from build123d import *

# Parameters (mm, degrees)
F2_DEPTH = 7.5
F3_DEPTH = 10


with BuildPart() as f2:
    # F1 (on Right) → F2 (new body, symmetric)
    with BuildSketch(Plane.YZ):
        Polygon((-9, 0), (0, 0), (10, 0), (10, 1), (-9, 7.5), align=None)
    extrude(amount=F2_DEPTH, both=True)

    # F0 (on Top) → F3 (cut, symmetric)
    with BuildSketch(Plane.XY):
        with BuildLine():
            ThreePointArc((-2.5, 0), (0, -2.5), (2.5, 0))
            Line((2.5, 0), (-2.5, 0))
        make_face()
        with BuildLine():
            Line((-2.5, 0), (2.5, 0))
            ThreePointArc((2.5, 0), (0, 2.5), (-2.5, 0))
        make_face()
    extrude(amount=F3_DEPTH, both=True, mode=Mode.SUBTRACT)


solid = f2.part
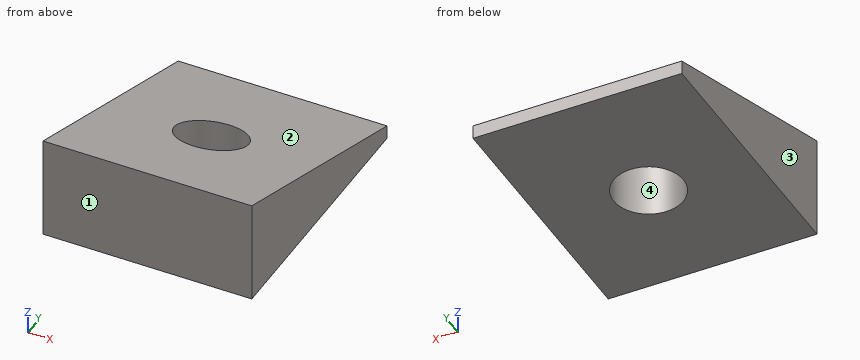
Model file for the job. Use its own axes, mm. Face numbers are marked on the shaded views. Coordinates: 2 decimals unless noted, no trailing zeros. Write each loop counter-clockwise with the first axis right and the second up, starting at its lowest first coordinate (ties: lowest second). Pieces come first, ordered by that corner, then holes. Notation, with made-up numbers: (-27, 49) -> (32, 49) arc R10 cw to (32, 62) -> close; hole circle Ø10 at (20.5, 60.25). An arc over 180 degrees is marked (long way). One line per item, written item: value. Start each with the question number.
1) Pull direction Y, two halves, no side cores. Call the marked faces 1, 2, 3 and 4: +Y half, -Y half, draft (parallel to the pull), parting line (faces both ways), or undercut.
2) Slice it at D-D on z = 6.5. Write the cut outline in (x, y), then the cut area to 3 significant figures.
3) Slice it at C-C on z = 3.5. Write the cut outline in (x, y), then the cut area to 3 significant figures.
4) Flat gauge pins, fed straight in: pin 1 Ø8 at (x, y) = (0, 0) entering from +Z; pin 2 Ø1.5 at (x, y) = (2.5, 7.5) entering from +Z; pin 3 Ø2 at (y, z) = (7.5, 2.5) entering from +X; pin 4 Ø6 at (x, y) = (4, 0.5) entering from +Z. Where does each tip first touch, or does it go through?
5) Slice it at B-B on y = 0. Write the cut outline in (x, z), then the cut area to 3 significant figures.
6) Probe probe 1 along X at (y, z) = (0, 3.1); probe 2 along Y at (x, z) = (-1.25, 0.5); probe 3 along X at (y, z) = (2, 3). List the from-to ranges inside material, lowest first.
7) Slice it at A-A on x = 2. Write the cut outline in (y, z), then the cut area to 3 significant figures.
Answers follow:
1. face 1: -Y half
1. face 2: +Y half
1. face 3: draft
1. face 4: undercut
2. outline: (-7.5, -9) -> (7.5, -9) -> (7.5, -6.08) -> (-7.5, -6.08) -> close
2. area: 43.8 mm2
3. outline: (-7.5, -9) -> (7.5, -9) -> (7.5, 2.69) -> (-7.5, 2.69) -> close; hole circle Ø5 at (0, 0)
3. area: 156 mm2
4. pin 1: z = 5.79
4. pin 2: z = 2.11
4. pin 3: x = 7.5
4. pin 4: z = 5.28
5. outline: (-7.5, 0) -> (-2.5, 0) -> (-2.5, 4.42) -> (-7.5, 4.42) -> close; (2.5, 0) -> (7.5, 0) -> (7.5, 4.42) -> (2.5, 4.42) -> close
5. area: 44.2 mm2
6. probe 1: -7.5 to -2.5, 2.5 to 7.5
6. probe 2: -9 to -2.17, 2.17 to 10
6. probe 3: -7.5 to -1.5, 1.5 to 7.5
7. outline: (-9, 0) -> (-1.5, 0) -> (-1.5, 4.93) -> (-9, 7.5) -> close; (1.5, 0) -> (10, 0) -> (10, 1) -> (1.5, 3.91) -> close
7. area: 67.5 mm2
